Here's how the part is built. I have some questions about the finished solid (model axes, mm). Face numbers are marked on the shaded views. A direction names the side the tool comes from. Give positions to 0.01 mm unless a question says otherwise; leave off trailing zeros. Loops run counter-clockwise (first coordinate to the right, second up) from the corner with the lowest first, then second, coordinate; pieces in that order, holes last.
Q1. Suppose I cut it at A-A (z = 0). List the corners of the cut face in (x, y) for me.
Q2. Thinking about a two-plate mould opening in Y: for the marked faces 3, 4 and 5, which applies, pulls with the +Y half, pulls with the -Y half, needs draft (parallel to the pull), parting line crosses it, or undercut?
Q3. For the marked faces 1 and 2, which set-ups out of +Z, -Z, +X, -X, +Y, -Y let a thin tool reach every point of the face, with its end or its side?
Q4. Suppose I cut it at B-B (x = 4). List the corners of the cut face in (y, z) for me.
Q5. I need wall thicknesses on probe 1 along X at (y, z) = (124.5, 0); probe 2 along Z at (x, y) = (-0.5, 20.5); probe 3 along X at (y, z) = (125, 4.5). Which ranges of each line are inside material? Lowest first, please.
Q6. I'm going to push flat-ended pins straight in: P1, Ø3, axis at y = 131, z = 10.5, coming from the -X side; P2, Ø1, axis at y = 45, z = 2, coming from the -X side; P3, Ø2, axis at y = 85.5, z = -2, coming from the -X side. Where does each tip first touch, or does it pass through?
```python
from build123d import *

# Parameters (mm, degrees)
SKETCH1_R           = 14.2875
SKETCH1_R_2         = 11.4125
BOSS_EXTRUDE1_DEPTH = 226.06
SKETCH2_W           = 28.575
SKETCH2_H           = 226.06
BOSS_EXTRUDE2_DEPTH = 12.7
BOSS_EXTRUDE3_DEPTH = 226.06
CUT_EXTRUDE1_DEPTH  = 29.575
FILLET1_R           = 8.5
FILLET2_R           = 8.5
FILLET3_R           = 1


with BuildPart() as part:
    # Sketch1 → Boss-Extrude1 (new body)
    with BuildSketch(Plane(origin=(0, 0, 0), x_dir=(1, 0, 0), z_dir=(0, 1, 0))):
        Circle(SKETCH1_R)
        Circle(SKETCH1_R_2, mode=Mode.SUBTRACT)
    extrude(amount=BOSS_EXTRUDE1_DEPTH)



with BuildPart() as body_2:
    # Sketch2 → Boss-Extrude2 (new body)
    with BuildSketch(Plane(origin=(14.2875, 0, 0), x_dir=(0, 0, -1), z_dir=(1, 0, 0))):
        with Locations((0, 113.03)):
            Rectangle(SKETCH2_W, SKETCH2_H)
    extrude(amount=BOSS_EXTRUDE2_DEPTH)


with BuildPart() as part_1:
    add(part.part)

    add(body_2.part)  # Boss-Extrude3 merges body 2
    # Sketch3 → Boss-Extrude3 (add, through all)
    with BuildSketch(Plane(origin=(0, 226.06, 0), x_dir=(1, 0, 0), z_dir=(0, 1, 0))):
        with BuildLine():
            Line((14.2875, -14.2875), (0, -14.2875))
            ThreePointArc((0, -14.2875), (14.2875, 0), (0, 14.2875))
            Line((0, 14.2875), (14.2875, 14.2875))
            Line((14.2875, 14.2875), (26.9875, 14.2875))
            Line((26.9875, 14.2875), (26.9875, -14.2875))
            Line((26.9875, -14.2875), (14.2875, -14.2875))
        make_face()
    extrude(amount=-BOSS_EXTRUDE3_DEPTH)

    # Sketch5 → Cut-Extrude1 (cut, through all)
    with BuildSketch(Plane.XY.offset(14.2875)):
        Polygon((26.9875, 226.06), (13.9875, 125.73), (13.9875, 100.33), (26.9875, 0), align=None)
    extrude(amount=-CUT_EXTRUDE1_DEPTH, mode=Mode.SUBTRACT)

    # Fillet1
    fillet1_edges = [part_1.edges().sort_by_distance(p)[0] for p in [
        (26.9875, 0, 0),
        (26.9875, 226.06, 0),
    ]]
    fillet(fillet1_edges, radius=FILLET1_R)

    # Fillet2
    fillet2_edges = [part_1.edges().sort_by_distance(p)[0] for p in [
        (13.9875, 125.73, 0),
        (13.9875, 100.33, 0),
    ]]
    fillet(fillet2_edges, radius=FILLET2_R)

    # Fillet3
    fillet3_edges = [part_1.edges().sort_by_distance(p)[0] for p in [
        (-14.2875, 0, 0),
        (8.657539107, 0, 14.2875),
        (8.657539107, 226.06, 14.2875),
        (19.901289107, 171.370804703, -14.2875),
        (8.657539107, 0, -14.2875),
        (8.657539107, 226.06, -14.2875),
        (23.69998215, 223.17097155, -14.2875),
        (23.69998215, 2.88902845, -14.2875),
        (19.901289107, 171.370804703, 14.2875),
        (23.69998215, 223.17097155, 14.2875),
        (23.69998215, 2.88902845, 14.2875),
        (19.901289107, 54.689195297, 14.2875),
        (19.901289107, 54.689195297, -14.2875),
        (13.9875, 113.03, 14.2875),
        (13.9875, 113.03, -14.2875),
        (14.005135098, 100.331137756, 14.2875),
        (14.005135098, 100.331137756, -14.2875),
        (14.005135098, 125.728862244, 14.2875),
        (14.005135098, 125.728862244, -14.2875),
        (-14.2875, 226.06, 0),
    ]]
    fillet(fillet3_edges, radius=FILLET3_R)


solid = part_1.part
```
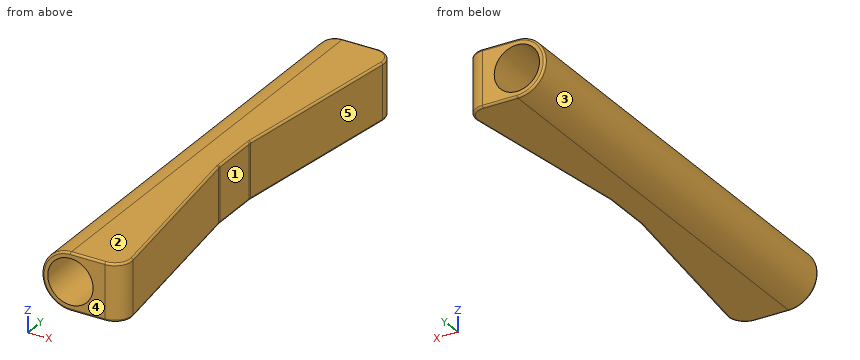
Solutions:
1. outline: (-14.29, 1) arc R1 ccw to (-13.29, 0) - (-11.41, 0) - (-11.41, 226.06) - (-13.29, 226.06) arc R1 ccw to (-14.29, 225.06) - close; (11.41, 0) - (17.32, 0) arc R8.5 ccw to (25.74, 9.59) - (14.06, 99.79) arc R8.5 cw to (13.99, 100.88) - (13.99, 125.18) arc R8.5 cw to (14.06, 126.27) - (25.74, 216.47) arc R8.5 ccw to (17.32, 226.06) - (11.41, 226.06) - close
2. face 3: needs draft
2. face 4: pulls with the -Y half
2. face 5: undercut
3. face 1: +Z, -Z, +X
3. face 2: +Z, +X, -X, +Y, -Y
4. outline: (0, -13.29) arc R1 ccw to (1, -14.29) - (225.06, -14.29) arc R1 ccw to (226.06, -13.29) - (226.06, -10.69) - (0, -10.69) - close; (0, 10.69) - (226.06, 10.69) - (226.06, 13.29) arc R1 ccw to (225.06, 14.29) - (1, 14.29) arc R1 ccw to (0, 13.29) - close
5. probe 1: x = -14.29 to -11.41, 11.41 to 13.99
5. probe 2: z = -14.28 to -11.4, 11.4 to 14.28
5. probe 3: x = -13.56 to -10.49, 10.49 to 13.99
6. P1: stops at x = -11.1
6. P2: stops at x = -14.21
6. P3: stops at x = -14.25
